from build123d import *

# Parameters (mm, degrees)
SKETCH1_W           = 15
SKETCH1_H           = 25
BOSS_EXTRUDE1_DEPTH = 5
SKETCH2_R           = 2.5
BOSS_EXTRUDE2_DEPTH = 5
FILLET1_R           = 7.5
SKETCH3_W           = 10
SKETCH3_H           = 10
BOSS_EXTRUDE3_DEPTH = 10
FILLET2_R           = 5
SKETCH4_R           = 2.5
CUT_EXTRUDE1_DEPTH  = 10
SKETCH5_W           = 25
SKETCH5_H           = 10
BOSS_EXTRUDE4_DEPTH = 15
SKETCH6_W           = 6
SKETCH6_H           = 15
CUT_EXTRUDE2_DEPTH  = 15
FILLET3_R           = 5
FILLET4_R           = 10
FILLET5_R           = 5


# Some blends are built 0.0001 mm under size
with BuildPart() as part:
    # Sketch1 → Boss-Extrude1 (new, symmetric)
    with BuildSketch(Plane.XY):
        Rectangle(SKETCH1_W, SKETCH1_H)
    extrude(amount=BOSS_EXTRUDE1_DEPTH, both=True)

    # Sketch2 → Boss-Extrude2 (add)
    with BuildSketch(Plane.XY.offset(5)):
        with BuildLine():
            ThreePointArc((-7.5, -20), (0, -27.5), (7.5, -20))
            Line((7.5, -20), (7.5, 20))
            ThreePointArc((7.5, 20), (0, 27.5), (-7.5, 20))
            Line((-7.5, 20), (-7.5, -20))
        make_face()
        with Locations((0, -20)):
            Circle(SKETCH2_R, mode=Mode.SUBTRACT)
        with Locations((0, 20)):
            Circle(SKETCH2_R, mode=Mode.SUBTRACT)
    boss_extrude2 = extrude(amount=BOSS_EXTRUDE2_DEPTH)

    # Mirror1: Boss-Extrude2 across plane
    add(boss_extrude2.mirror(Plane.XY))

    # Fillet1
    fillet1_edges = [part.edges().sort_by_distance(p)[0] for p in [
        (7.5, -12.5, 0),
        (-7.5, -12.5, 0),
        (-7.5, 12.5, 0),
        (7.5, 12.5, 0),
    ]]
    fillet(fillet1_edges, radius=FILLET1_R - 0.0001)  # a hair under: the kernel refuses the full size

    # Sketch3 → Boss-Extrude3 (add)
    with BuildSketch(Plane(origin=(7.5, 0, 0), x_dir=(0, 0, -1), z_dir=(1, 0, 0))):
        Rectangle(SKETCH3_W, SKETCH3_H)
    extrude(amount=BOSS_EXTRUDE3_DEPTH)

    # Fillet2
    fillet2_edges = [part.edges().sort_by_distance(p)[0] for p in [
        (17.5, 0, 5),
        (17.5, 0, -5),
    ]]
    fillet(fillet2_edges, radius=FILLET2_R - 0.0001)  # a hair under: the kernel refuses the full size

    # Sketch4 → Cut-Extrude1 (cut)
    with BuildSketch(Plane(origin=(0, 5, 0), x_dir=(1, 0, 0), z_dir=(0, 1, 0))):
        with Locations(Location((12.5, 0, 0), (0, 0, 270))):
            Circle(SKETCH4_R)
    extrude(amount=-CUT_EXTRUDE1_DEPTH, mode=Mode.SUBTRACT)

    # Sketch5 → Boss-Extrude4 (add)
    with BuildSketch(Plane.ZY.offset(7.5)):
        Rectangle(SKETCH5_W, SKETCH5_H)
    extrude(amount=BOSS_EXTRUDE4_DEPTH)

    # Sketch6 → Cut-Extrude2 (cut)
    with BuildSketch(Plane.XZ.offset(5)):
        with Locations((-15, 0)):
            Rectangle(SKETCH6_W, SKETCH6_H)
    extrude(amount=-CUT_EXTRUDE2_DEPTH, mode=Mode.SUBTRACT)

    # Fillet3
    # the kernel refuses this fillet: 5 mm, written as the material it adds along each edge
    with BuildSketch(Plane(origin=(-7.5, 5, 10), x_dir=(1, 0, 0), z_dir=(0, -1, 0))) as fillet3_piece_1:
        with BuildLine():
            CenterArc((4.330127019, 5), FILLET3_R, 210, 60)
            Line((0, 2.5), (0, 0))
            Line((0, 0), (4.330127019, 0))
        make_face()
    extrude(amount=10)
    with BuildSketch(Plane(origin=(-7.5, 5, -10), x_dir=(1, 0, 0), z_dir=(0, -1, 0))) as fillet3_piece_2:
        with BuildLine():
            CenterArc((4.330127019, -5), FILLET3_R, 90, 60)
            Line((0, -2.5), (0, 0))
            Line((0, 0), (4.330127019, 0))
        make_face()
    extrude(amount=10)

    # Fillet4
    fillet4_edges = [part.edges().sort_by_distance(p)[0] for p in [
        (-7.5, 0, 12.5),
        (-7.5, 0, -12.5),
        (-22.5, 0, 12.5),
        (-22.5, 0, -12.5),
    ]]
    fillet(fillet4_edges, radius=FILLET4_R)

    # Fillet5
    fillet5_edges = [part.edges().sort_by_distance(p)[0] for p in [
        (-18, 0, -7.5),
        (-18, 0, 7.5),
    ]]
    fillet(fillet5_edges, radius=FILLET5_R)


solid = part.part
For this review, take the finished solid that the model builds, in its own axes (mm). A direction names the side the tool comes from. Coordinates: 2 decimals unless noted, no trailing zeros. Loops run counter-clockwise (first coordinate to the right, second up) from the corner with the lowest first, then second, coordinate; pieces in that order, holes last. Notation, with made-up numbers: (-8, -2.5) - (35, -2.5) arc R26 cw to (35, 31.5) - close; hole circle Ø2 at (-1, 47.25). An arc over 180 degrees is marked (long way). Use a Markdown table: item, result. Add a question column.
Item 1: We need section C-C (z = -8.25). Give the boundary of the cut face in (x, y).
Item 2: We need section A-A (y = 2.5). Give the number of separate pieces and of enclosed holes in the cut face, and give its area (3 significant figures).
Item 3: For line 1 (X direction, y = 1.25, z = 0); line 2 (Y direction, x = 0, z = 9); line 3 (Z direction, x = 3.5, y = -13), list the stretches that pass through material, from the lowest coordinate up.
Item 4: Mouldability with a two-part tool opening along Z and no side actions: class faces 5 (the face through (-8.535, 0.07, 12.062)), 6 (the face through (0.16, 27.5, 7.46)), 7 (the face through (-16.5, 0.07, 6.07)) as pulls with the +Z half, pulls with the -Z half, needs draft (parallel to the pull), parting line crosses it, or undercut.
Item 5: We need section B-B (y = 16). Give the boundary of the cut face in (x, z), and give its area (3 significant figures).
Item 6: We need section D-D (x = -16). Give the boundary of the cut face in (y, z), and give its area (3 significant figures).
Item 7: Tool access review of faces 1 (the face through (10, 0, 5)), 2 (the face through (-18, 0, 0)), 3 (the face through (10, -5, -1)), 4 (the face through (5.361, -10.245, 0.07)): name each direction out of +Z, -Z, +X, -X, +Y, -Y from which nothing blocks a thin tool from reaching the whole face with its end or side.
Item 8: Insertion check: pin 1 Ø2 at (x, y) = (9, -0.5) entering from +Z; pin 2 Ø11 at (x, z) = (14, -2.5) entering from -Y; pin 3 Ø4 at (y, z) = (0.5, -8) entering from +X. Each pin has a flat end and moves straight along its axis. Give the tip position at first contact, or say it passes through.
Results list:
| question | item | result |
|---|---|---|
| 1 | outline | (-20.68, -5) - (-7.5, -5) - (-7.5, -20) arc R7.5 ccw to (7.5, -20) - (7.5, 20) arc R7.5 ccw to (-7.5, 20) - (-7.5, 5) - (-20.68, 5) - close; hole circle Ø5 at (0, -20); hole circle Ø5 at (0, 20) |
| 2 | separate pieces | 1 |
| 2 | enclosed holes | 2 |
| 2 | area | 626 mm^2 |
| 3 | line 1 | x = -22.5 to -18, -12 to 10, 15 to 17.5 |
| 3 | line 2 | y = -27.5 to -22.5, -17.5 to 17.5, 22.5 to 27.5 |
| 3 | line 3 | z = -10 to -5, 5 to 10 |
| 4 | face 5 | pulls with the +Z half |
| 4 | face 6 | needs draft |
| 4 | face 7 | undercut |
| 5 | outline | (-7.5, -10) - (7.5, -10) - (7.5, -5) - (-7.5, -5) - close; (-7.5, 5) - (7.5, 5) - (7.5, 10) - (-7.5, 10) - close |
| 5 | area | 150 mm^2 |
| 6 | outline | (-5, -11.87) - (5, -11.87) - (5, -6.5) - (-5, -6.5) - close; (-5, 6.5) - (5, 6.5) - (5, 11.87) - (-5, 11.87) - close |
| 6 | area | 107 mm^2 |
| 7 | face 1 | +Z, +X, +Y, -Y |
| 7 | face 2 | +Y, -Y |
| 7 | face 3 | +Z, -Z, +X, -Y |
| 7 | face 4 | +X, -Y |
| 8 | pin 1 | stops at z = 5 |
| 8 | pin 2 | stops at y = -5 |
| 8 | pin 3 | stops at x = 7.5 |
